Source: three-view drawing plus pictorial views. Frame: mm from the lowest corner of the part. A direction names the side the tool comes from. Coordinates: 2 decimals unless noted, no trailing zeros. Loops run counter-clockwise (first coordinate to the right, second up) from the corner with the lowest first, then second, coordinate; pieces in that order, holes last. Notation, with made-up numbers: (-29, 45.5) - (-19, 45.5) arc R23 ccw to (-19, 79.5) - close; hole circle Ø9 at (26, 79). An arc over 180 degrees is marked (long way). Return JSON: item names as keys, results as strings.
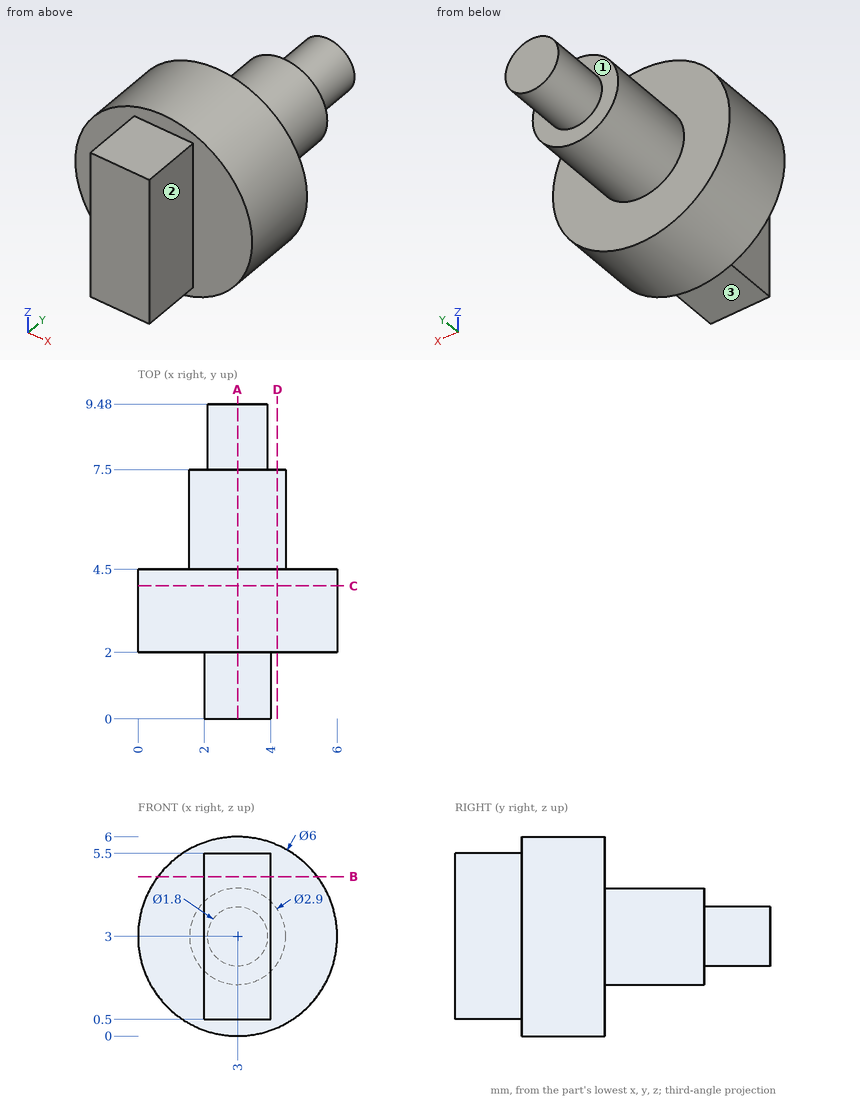
Item 1: Section query D-D, the plane x = 4.2. Return loops of the section in (y, z).
Worked out:
{"outline": "(2, 0.25) - (4.5, 0.25) - (4.5, 2.19) - (7.5, 2.19) - (7.5, 3.81) - (4.5, 3.81) - (4.5, 5.75) - (2, 5.75) - close"}
Item 2: Section query A-A, the plane x = 3. Return loops of the section in (y, z).
Worked out:
{"outline": "(0, 0.5) - (2, 0.5) - (2, 0) - (4.5, 0) - (4.5, 1.55) - (7.5, 1.55) - (7.5, 2.1) - (9.48, 2.1) - (9.48, 3.9) - (7.5, 3.9) - (7.5, 4.45) - (4.5, 4.45) - (4.5, 6) - (2, 6) - (2, 5.5) - (0, 5.5) - close"}
Item 3: Section query B-B, the plane z = 4.8. Return loops of the section in (x, y).
Worked out:
{"outline": "(0.6, 2) - (2, 2) - (2, 0) - (4, 0) - (4, 2) - (5.4, 2) - (5.4, 4.5) - (0.6, 4.5) - close"}
Item 4: Section query C-C, the plane y = 4. Return loops of the section in (x, z), and give its area (3 significant figures).
Worked out:
{"outline": "circle Ø6 at (3, 3)", "area": "28.3 mm^2"}
Item 5: Ray query, probe 1 along Y at (x, z) = (4.1, 1.7); probe 2 along Y at (x, z) = (2.5, 4.1); probe 3 along X at (y, z) = (0.5, 1.75). Return the intervals inside material, ascending. Write a range as from..to.
Worked out:
{"probe 1": "2..4.5", "probe 2": "0..7.5", "probe 3": "2..4"}
Item 6: Reachability of the marked faces 1, 2 and 3 from +Z, -Z, +X, -X, +Y, -Y: full face, straight path, thin tool, end or side. Return the list, or none.
Worked out:
{"face 1": "+Y", "face 2": "+Z, -Z, +X, -Y", "face 3": "-Z, +X, -X, -Y"}
Item 7: First-contact query: pin 1 Ø3 at (x, y) = (4.5, 6.5) entering from -Z; pin 2 Ø1 at (x, y) = (3, 1) entering from -Z; pin 3 Ø0.6 at (x, y) = (3.5, 1) entering from +Z; pin 4 Ø1.5 at (x, y) = (2.5, 4) entering from -Z. Flat tips, straight axial feed; report the tip coordinate or a pass-through.
Worked out:
{"pin 1": "z = 1.55", "pin 2": "z = 0.5", "pin 3": "z = 5.5", "pin 4": "z = 0"}
